```python
from build123d import *

# Parameters (mm, degrees)
F0_R     = 10
F0_R_2   = 2.5
F1_DEPTH = 5
F2_R     = 5
F2_R_2   = 2.5
F3_DEPTH = 30
F4_R     = 2.49999


# Not quite as in the source:
# - a fillet or chamfer is up to 0.001 mm smaller than in the source, because OpenCascade refuses the exact size


with BuildPart() as f1:
    # F0 (on Top) → F1 (new body)
    with BuildSketch(Plane.XY):
        Circle(F0_R)
        Circle(F0_R_2, mode=Mode.SUBTRACT)
    extrude(amount=F1_DEPTH)

    # F2 (on face) → F3 (join)
    with BuildSketch(Plane(origin=(0, 0, 0), x_dir=(1, 0, 0), z_dir=(0, 0, -1))):
        Circle(F2_R)
        Circle(F2_R_2, mode=Mode.SUBTRACT)
    extrude(amount=F3_DEPTH)

    # F4 (radius 2.5 in the source; OpenCascade refuses exactly that, so slightly less here)
    f4_edges = [f1.edges().sort_by_distance(p)[0] for p in [
        (-10, 0, 5),
        (-2.5, 0, 5),
        (-2.5, 0, -30),
    ]]
    fillet(f4_edges, radius=F4_R)


solid = f1.part
```
Read the model definition and answer for the solid it produces. Units are mm, in the model's axes. A direction names the side the tool comes from. Give positions to 0.01 mm unless a question says otherwise; leave off trailing zeros. Write each loop counter-clockwise with the first axis right and the second up, starting at its lowest first coordinate (ties: lowest second). Pieces come first, ordered by that corner, then holes. Notation, with made-up numbers: (-13.5, 76) -> (33.5, 76) arc R31 ccw to (33.5, 101) -> close; hole circle Ø8 at (22.5, 72.5). An arc over 180 degrees is marked (long way). Answer in a Markdown table with one row per item.
1) Each of these flat-tipped pins is pushed along its axis until it touches: pin 1 Ø5 at (y, z) = (-6, -4) entering from -X; pin 2 Ø1 at (x, z) = (-6.5, -18.5) entering from -Y; pin 3 Ø2 at (x, y) = (-4.5, 7.5) entering from -Z; pin 4 Ø8 at (x, y) = (0, 0) entering from +Z. Where does it stop, or does it pass through?
Results list:
| item | result |
|---|---|
| pin 1 | x = -3.57 |
| pin 2 | through |
| pin 3 | z = 0 |
| pin 4 | z = 4.79 |
2) Determine the mould class of faces 3 (the cylindrical face through (-1.08, 4.88, -14.79)), 4 (the flat face through (5, -2, 5)), 5 (the cylindrical face through (-0.54, 2.44, -12.29)) for opening direction X: released by +X, released by -X, zero draft, split by the parting line, or undercut.
Results list:
| item | result |
|---|---|
| face 3 | split by the parting line |
| face 4 | zero draft |
| face 5 | undercut |
3) Straight lines are drawn through the part: line 1 (X direction, y = 0, z = -15); line 2 (Z direction, x = -5, y = -3.5). For each, find the intervals that lie inside material, in ascending order. Write a range as [from, to].
Results list:
| item | result |
|---|---|
| line 1 | [-5, -2.5], [2.5, 5] |
| line 2 | [0, 5] |
4) Section C-C on z = -1.5 is taken. Give the vertices of the cut face in (x, y), plus the area to 3 significant figures.
Results list:
| item | result |
|---|---|
| outline | circle Ø10 at (0, 0); hole circle Ø5 at (0, 0) |
| area | 58.9 mm^2 |
5) A tool of negligible diameter and unlimited length cuts with its end or side. For faces 1 (the cylindrical face through (-2.17, -9.76, 1.23)), 2 (the flat face through (-5, -2, 0)), from which of +Z, -Z, +X, -X, +Y, -Y can it reach the whole face along a straight path? Write none if from no direction.
Results list:
| item | result |
|---|---|
| face 1 | +Z, -Z |
| face 2 | -Z |
